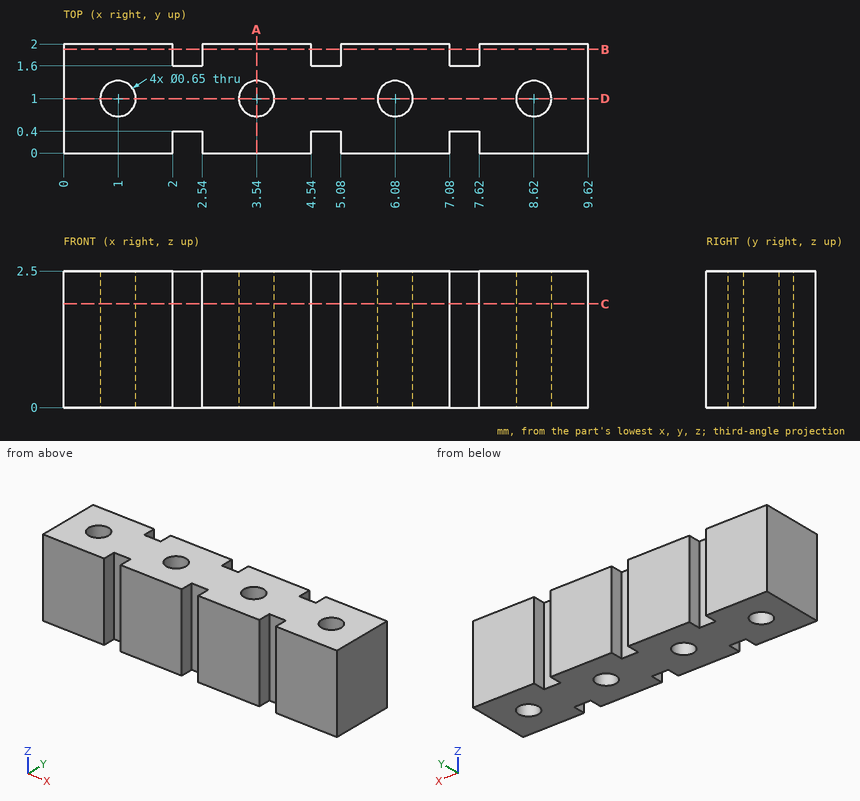
Could you check a few things on this drawing? It's one solid part, dimensions in mm from its lowest x, y, z. Give positions to 0.01 mm unless a question says otherwise; leave off trailing zeros. Order: outer loops, then holes, each group sorted by start corner. A loop starts at its lowest first (then second) coordinate and runs counter-clockwise, first axis right, second up. Notation, with made-up numbers: (-13.75, 60.25) - (13.25, 60.25) arc R32 ccw to (13.25, 88.25) - close; hole circle Ø5 at (61.25, -8.75). An arc over 180 degrees is marked (long way). One line per question, with ' | ' between items. Start each with the question number.
Item 1: I want a section at B-B on y = 1.9. Write out the boundary of the cut face in (x, z).
Item 2: I want a section at A-A on x = 3.54. Write out the boundary of the cut face in (y, z) (3 decimals), then the cut area to 4 significant figures.
Item 3: I want a section at C-C on z = 1.9. Give the number of separate pieces and of enclosed holes in the cut face, then the cut area to 3 significant figures.
Item 4: I need wall thicknesses on probe 1 along X at (y, z) = (1.8, 0.4); probe 2 along X at (y, z) = (1.15, 0.85); probe 3 along Y at (x, z) = (6.08, 1.7) (3 decimals). Which ranges of each line are inside material? Lowest first, please. Write a range as [from, to].
Item 5: I want a section at D-D on y = 1. Write out the boundary of the cut face in (x, z) (3 decimals).
Verdict:
1) outline: (0, 0) - (2, 0) - (2, 2.5) - (0, 2.5) - close; (2.54, 0) - (4.54, 0) - (4.54, 2.5) - (2.54, 2.5) - close; (5.08, 0) - (7.08, 0) - (7.08, 2.5) - (5.08, 2.5) - close; (7.62, 0) - (9.62, 0) - (9.62, 2.5) - (7.62, 2.5) - close
2) outline: (0, 0) - (0.675, 0) - (0.675, 2.5) - (0, 2.5) - close; (1.325, 0) - (2, 0) - (2, 2.5) - (1.325, 2.5) - close | area: 3.375 mm^2
3) separate pieces: 1 | enclosed holes: 4 | area: 16.6 mm^2
4) probe 1: [0, 2], [2.54, 4.54], [5.08, 7.08], [7.62, 9.62] | probe 2: [0, 0.71], [1.29, 3.25], [3.83, 5.79], [6.37, 8.33], [8.91, 9.62] | probe 3: [0, 0.675], [1.325, 2]
5) outline: (0, 0) - (0.675, 0) - (0.675, 2.5) - (0, 2.5) - close; (1.325, 0) - (3.215, 0) - (3.215, 2.5) - (1.325, 2.5) - close; (3.865, 0) - (5.755, 0) - (5.755, 2.5) - (3.865, 2.5) - close; (6.405, 0) - (8.295, 0) - (8.295, 2.5) - (6.405, 2.5) - close; (8.945, 0) - (9.62, 0) - (9.62, 2.5) - (8.945, 2.5) - close
